CAD build for the part. Positions are in the model's coordinates, mm. Coordinates: 2 decimals unless noted, no trailing zeros. Write each loop counter-clockwise with the first axis right and the second up, starting at its lowest first coordinate (ties: lowest second). Pieces come first, ordered by that corner, then holes. Notation, with made-up numbers: (72.5, -34.5) -> (114.5, -34.5) arc R32 ccw to (114.5, -8.5) -> close; hole circle Ø10 at (42, -12.5). An arc over 180 degrees is marked (long way). Answer as CSV lines item,"result".
Autodesk Inventor part; units mm, degrees
ref_plane "YZ Plane" through (0, 0, 0) normal (1, 0, 0) x (0, 1, 0)
ref_plane "XZ Plane" through (0, 0, 0) normal (0, 1, 0) x (-1, 0, 0)
ref_plane "XY Plane" through (0, 0, 0) normal (0, 0, 1) x (1, 0, 0)
sketch "Sketch2" plane through (0, 0, 0) normal (0, 0, 1) x (1, 0, 0)
  line L0 (-53, -96) -> (53, -96)
  line L1 (53, -96) -> (53, 96)
  line L2 (53, 96) -> (-53, 96)
  line L3 (-53, 96) -> (-53, -96)
  line L4 (-53, -96) -> (53, 96) construction
  line L5 (53, -96) -> (-53, 96) construction
  line L6 (-103, -146) -> (103, -146)
  line L7 (103, -146) -> (103, 146)
  line L8 (103, 146) -> (-103, 146)
  line L9 (-103, 146) -> (-103, -146)
  point P0 (0, 0)
  dimension "d31" = 50
  dimension "d60" = 192
  dimension "d61" = 106
extrude "Plate2" add sketch "Sketch2" along normal blind 8 contours L3 L2 L1 L0 | L9 L8 L7 L6
sketch "Sketch5" plane through (0, 0, 8) normal (0, 0, 1) x (1, 0, 0)
  line L0 (103, -146) -> (-103, -146) construction
  line L1 (103, 146) -> (103, -146) construction
  line L2 (-103, 146) -> (103, 146) construction
  line L3 (-103, -146) -> (-103, 146) construction
  line L4 (-84, 127) -> (84, 127) construction
  line L5 (84, 127) -> (84, -127) construction
  line L6 (84, -127) -> (-84, -127) construction
  line L7 (-84, -127) -> (-84, 127) construction
  line L8 (-28, -127) -> (28, -127)
  line L9 (28, -127) -> (28, 127) construction
  line L10 (28, 127) -> (-28, 127)
  line L11 (-28, 127) -> (-28, -127) construction
  line L12 (-28, 0) -> (28, 0) construction
  point P0 (0, 0)
  point P1 (0, -127)
  point P2 (-84, -63.5)
  point P3 (-84, 0)
  point P4 (-84, 63.5)
  point P5 (84, 63.5)
  point P6 (84, 0)
  point P7 (84, -63.5)
  point P8 (0, 0)
  dimension "d34" = 19
  dimension "d47" = 63.5
  dimension "d48" = 63.5
  dimension "d49" = 56
  dimension "d50" = 56
fillet "Corner Round1" radius 6 4 edges at (-103, -146, 4) (-103, 146, 4) (103, 146, 4) (103, -146, 4)
hole "Hole1" at (-84, -127, 8) at (-84, -63.5, 8) at (-84, 0, 8) at (-84, 63.5, 8) at (-84, 127, 8) at (84, 127, 8) at (84, 63.5, 8) at (84, 0, 8) at (84, -63.5, 8) at (84, -127, 8) at (-28, -127, 8) at (28, 127, 8) at (28, -127, 8) at (-28, 127, 8) direction (0, 0, -1) diameter 17 end through all
equation "\"d60\" = ChargingHatch_width - 2 * Thickness"
equation "\"d61\" = ChargingHatch_hight - 2 * Thickness"
equation "\"d56\" = Thickness"
equation "\"d14\" = Thickness"
equation "\"BendReliefWidth\" = Thickness"
equation "\"BendReliefDepth\" = 0.5 * Thickness"
equation "\"CornerReliefSize\" = 4 * Thickness"
equation "\"MinimumRemnant\" = 2 * Thickness"
equation "\"TransitionRadius\" = BendRadius"
equation "\"JacobiRadiusSize\" = BendRadius"
equation "\"GapSize\" = Thickness"
properties part number "PRS 9607 charging flange rect_D1200 940" material "Steel"
Item 1: Flat gauge pin, fed straight in: pin 1 (12 mm diameter, centred on x = 61, y = -92, fed in from -Z). Where does the tip first touch, or does it go through?
Answer below:
pin 1,"stops at z = 0"
Item 2: Two-plate mould, pull along X, no slides. Class faces 1 (the cylindrical face through (101.196, -144.289, 4.056)), 2 (the cylindrical face through (-101.196, 144.289, 4.056)), 3 (the cylindrical face through (31.26, -134.85, 3.94)): pulls with the +X half, pulls with the -X half, needs draft (parallel to the pull), parting line crosses it, or undercut.
Answer below:
face 1,"pulls with the +X half"
face 2,"pulls with the -X half"
face 3,"undercut"
Item 3: Saw through at C-C on z = 1.5. State how many separate pieces and enclosed holes the cut face has, and give its area (3 significant figures).
Answer below:
separate pieces,"1"
enclosed holes,"14"
area,"56,900 mm2"
Item 4: Saw through at A-A on y = 0. Give the cut face in (x, z), and give its area (3 significant figures).
Answer below:
outline,"(-103, 0) -> (-92.5, 0) -> (-92.5, 8) -> (-103, 8) -> close; (-75.5, 0) -> (75.5, 0) -> (75.5, 8) -> (-75.5, 8) -> close; (92.5, 0) -> (103, 0) -> (103, 8) -> (92.5, 8) -> close"
area,"1,380 mm2"
Item 5: Saw through at D-D on y = -127. Give the cut face in (x, z), and give its area (3 significant figures).
Answer below:
outline,"(-103, 0) -> (-92.5, 0) -> (-92.5, 8) -> (-103, 8) -> close; (-75.5, 0) -> (-36.5, 0) -> (-36.5, 8) -> (-75.5, 8) -> close; (-19.5, 0) -> (19.5, 0) -> (19.5, 8) -> (-19.5, 8) -> close; (36.5, 0) -> (75.5, 0) -> (75.5, 8) -> (36.5, 8) -> close; (92.5, 0) -> (103, 0) -> (103, 8) -> (92.5, 8) -> close"
area,"1,100 mm2"
Item 6: Saw through at B-B on x = 32. Give the cut face in (y, z), and give its area (3 significant figures).
Answer below:
outline,"(-146, 0) -> (-134.5, 0) -> (-134.5, 8) -> (-146, 8) -> close; (-119.5, 0) -> (119.5, 0) -> (119.5, 8) -> (-119.5, 8) -> close; (134.5, 0) -> (146, 0) -> (146, 8) -> (134.5, 8) -> close"
area,"2,100 mm2"
Item 7: Wall check: line 1 (X direction, y = -63.5, z = 6); line 2 (Y direction, x = -28, z = 6.25); line 3 (Y direction, x = 84, z = 2). Give the ranges that are in metal, low to high. Write a range as from..to.
Answer below:
line 1,"x = -103..-92.5, -75.5..75.5, 92.5..103"
line 2,"y = -146..-135.5, -118.5..118.5, 135.5..146"
line 3,"y = -146..-135.5, -118.5..-72, -55..-8.5, 8.5..55, 72..118.5, 135.5..146"
